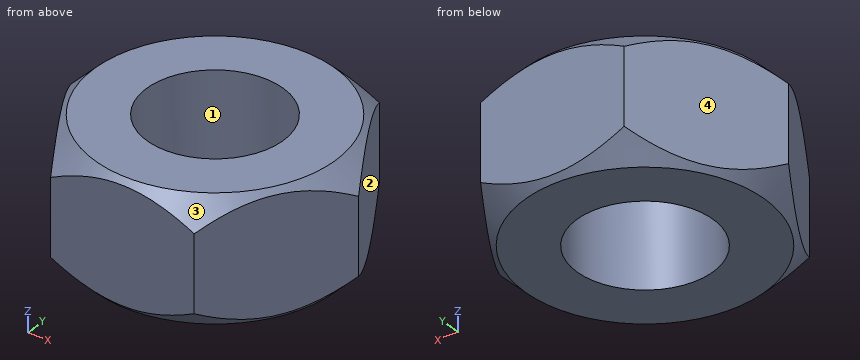
from build123d import *

# Parameters (mm, degrees)
BOSS_EXTRUDE1_DEPTH             = 6.4
TAP_DRILL_FOR_M8X1_0_TAP1_D     = 7
TAP_DRILL_FOR_M8X1_0_TAP1_DEPTH = 16


with BuildPart() as part:
    # Sketch1 → Boss-Extrude1 (new body)
    with BuildSketch(Plane.XY):
        Polygon((7.418950959, 0), (3.70947548, 6.425), (-3.70947548, 6.425), (-7.418950959, 0), (-3.70947548, -6.425), (3.70947548, -6.425), align=None)
    extrude(amount=BOSS_EXTRUDE1_DEPTH)

    # Tap Drill for M8x1.0 Tap1
    with Locations(Plane(origin=(0, 0, 0), x_dir=(-1, 0, 0), z_dir=(0, 0, -1))):
        with Locations((0, 0)):
            Hole(TAP_DRILL_FOR_M8X1_0_TAP1_D / 2, depth=TAP_DRILL_FOR_M8X1_0_TAP1_DEPTH)

    # Sketch4 → Cut-Revolve1 (revolve, cut)
    with BuildSketch(Plane(origin=(0, 0, 0), x_dir=(-1, 0, 0), z_dir=(0, -1, 0))):
        Polygon((-7.418950959, 0), (-7.418950959, -1.25), (-6.168950959, 0), align=None)
        Polygon((-7.418950959, -6.4), (-7.418950959, -5.15), (-6.168950959, -6.4), align=None)
    revolve(axis=Axis((0, 0, 6.4), (0, 0, -1)), mode=Mode.SUBTRACT)


solid = part.part
Design review of the part built by this model. Coordinates are the model's own, in mm. Face numbers are marked on the shaded views. Round coordinates to 2 decimals unless told otherwise and drop trailing zeros. Write each loop counter-clockwise with the first axis right and the second up, starting at its lowest first coordinate (ties: lowest second). Pieces come first, ordered by that corner, then holes. Notation, with made-up numbers: (46.25, 52) - (75.25, 52) arc R8 cw to (75.25, 60) - close; hole circle Ø10 at (-37.5, 49). An arc over 180 degrees is marked (long way). Return JSON: item names as keys, results as strings. Group by question number.
Item 1: Insertion check: P1, Ø1.5, axis at y = 4, z = 4.5, coming from the +X side; P2, Ø4, axis at x = 2.5, y = -3, coming from the -Z side. Each pin has a flat end and moves straight along its axis. Give the tip position at first contact, or say it passes through.
Item 2: For probe 1 along Y at (x, z) = (0, 4.5) (3 decimals); probe 2 along Y at (x, z) = (-1.75, 2) (3 decimals); probe 3 along X at (y, z) = (1.5, 4.75), list the stretches that pass through material, from the lowest coordinate up. Write a range as [from, to].
Item 3: We need section B-B on z = 4.75. Write out the cut boundary in (x, y) (3 decimals).
Item 4: We need section A-A on x = 0. Write out the cut boundary in (y, z) (3 decimals).
Item 5: We need section C-C on z = 0.5. Write out the cut boundary in (x, y) (3 decimals), and give its area (3 significant figures).
Item 6: The part is to be moulded in two halves that separate along X. For the marked faces 1, 2, 3 and 4, say which applies: pulls with the +X half, pulls with the -X half, needs draft (parallel to the pull), parting line crosses it, or undercut.
Model answer:
{
 "1": {"P1": "stops at x = 5.54", "P2": "stops at z = 0"},
 "2": {"probe 1": "y = [-6.425, -3.5], [3.5, 6.425]", "probe 2": "y = [-6.425, -3.031], [3.031, 6.425]", "probe 3": "x = [-6.55, -3.16], [3.16, 6.55]"},
 "3": {"outline": "(-7.419, 0) - (-3.709, -6.425) - (3.709, -6.425) - (7.419, 0) - (3.709, 6.425) - (-3.709, 6.425) - close; hole circle Ø7 at (0, 0)"},
 "4": {"outline": "(-6.425, 0.256) - (-6.169, 0) - (-3.5, 0) - (-3.5, 6.4) - (-6.169, 6.4) - (-6.425, 6.144) - close; (3.5, 0) - (6.169, 0) - (6.425, 0.256) - (6.425, 6.144) - (6.169, 6.4) - (3.5, 6.4) - close"},
 "5": {"outline": "(-6.458, -1.665) - (-4.671, -4.76) arc R6.669 ccw to (-1.787, -6.425) - (1.787, -6.425) arc R6.669 ccw to (4.671, -4.76) - (6.458, -1.665) arc R6.669 ccw to (6.458, 1.665) - (4.671, 4.76) arc R6.669 ccw to (1.787, 6.425) - (-1.787, 6.425) arc R6.669 ccw to (-4.671, 4.76) - (-6.458, 1.665) arc R6.669 ccw to start; hole circle Ø7 at (0, 0)", "area": "97.7 mm²"},
 "6": {"face 1": "undercut", "face 2": "pulls with the +X half", "face 3": "parting line crosses it", "face 4": "pulls with the -X half"}
}
